```python
from build123d import *

# Parameters (mm, degrees)
SKETCH1_W                  = 85.725
SKETCH1_H                  = 38.1
BOSS_EXTRUDE1_DEPTH        = 12.7
F_1_2_0_5_DIAMETER_HOLE1_D = 12.7
F_1_4_CLEARANCE_HOLE1_D    = 6.7564


with BuildPart() as part:
    # Sketch1 → Boss-Extrude1 (new, symmetric)
    with BuildSketch(Plane(origin=(0, 0, 0), x_dir=(1, 0, 0), z_dir=(0, 1, 0))):
        Rectangle(SKETCH1_W, SKETCH1_H)
    extrude(amount=BOSS_EXTRUDE1_DEPTH, both=True)

    # 1/2 (0.5) Diameter Hole1 (through all)
    with Locations(Plane.XY.offset(19.05)):
        with Locations((30.1625, 0)):
            Hole(F_1_2_0_5_DIAMETER_HOLE1_D / 2)

    # 1/4 Clearance Hole1 (through all)
    with Locations(Plane(origin=(0, 12.7, 0), x_dir=(1, 0, 0), z_dir=(0, 1, 0))):
        with Locations((-33.3375, 0), (-1.5875, 0)):
            Hole(F_1_4_CLEARANCE_HOLE1_D / 2)


solid = part.part
```
Geometry: final body of the model. Coordinates: model frame, mm. Round coordinates to 2 decimals unless told otherwise and drop trailing zeros. Write each loop counter-clockwise with the first axis right and the second up, starting at its lowest first coordinate (ties: lowest second). Pieces come first, ordered by that corner, then holes. Notation, with made-up numbers: M 45.5,-20 L 101.5,-20 A29 cw 101.5,5 Z; hole C -32,9.25 d7. An arc over 180 degrees is marked long. Answer in a Markdown table with one row per item. Add a question column.
(1) Cut plane A-A, the plane y = 0. Return the cut outline in (x, z), then the cut area to 3 significant figures.
(2) Contact query for a flat-ended pin moving along its axis: pin 1 (4 mm diameter, centred on x = 26.5, y = 4, fed in from +Z). Output: stop coordinate, or through.
(3) Ray query, L1, parallel to X at y = 2, z = -0.5; L2, parallel to X at y = 5, z = 1; L3, parallel to X at y = -11.25, z = -1. Return the intervals inside material, ascending.
(4) Cut plane D-D, the plane z = 16.5. Return the cut outline in (x, y).
(5) Cut plane B-B, the plane z = 0. Return the cut outline in (x, y), then the cut area to 3 significant figures.
(6) Cut plane C-C, the plane y = -10.25. Return the cut outline in (x, z).
(7) Draft query along X for faces 1 (the face through (-1, -12.7, -5)), 2 (the face through (-0.86, -0.18, 3.3)), 3 (the face through (-42.862, 0, 0)), 4 (the face through (-29.963, -0.178, -0.149)). Return one class per face: pulls with the +X half, pulls with the -X half, needs draft (parallel to the pull), parting line crosses it, or undercut.
Established:
| question | item | result |
|---|---|---|
| 1 | outline | M -42.86,-19.05 L 23.81,-19.05 L 23.81,19.05 L -42.86,19.05 Z; M 36.51,-19.05 L 42.86,-19.05 L 42.86,19.05 L 36.51,19.05 Z; hole C -33.34,0 d6.76; hole C -1.59,0 d6.76 |
| 1 | area | 2,710 mm² |
| 2 | pin 1 | z = 19.05 |
| 3 | L1 | -42.86 to -36.68, -30 to -4.93, 1.75 to 24.14, 36.19 to 42.86 |
| 3 | L2 | -42.86 to -36.56, -30.11 to -4.81, 1.64 to 26.25, 34.08 to 42.86 |
| 3 | L3 | -42.86 to -36.56, -30.11 to -4.81, 1.64 to 42.86 |
| 4 | outline | M -42.86,-12.7 L 42.86,-12.7 L 42.86,12.7 L -42.86,12.7 Z; hole C 30.16,0 d12.7 |
| 5 | outline | M -42.86,-12.7 L -36.72,-12.7 L -36.72,12.7 L -42.86,12.7 Z; M -29.96,-12.7 L -4.97,-12.7 L -4.97,12.7 L -29.96,12.7 Z; M 1.79,-12.7 L 42.86,-12.7 L 42.86,12.7 L 1.79,12.7 Z; hole C 30.16,0 d12.7 |
| 5 | area | 1,710 mm² |
| 6 | outline | M -42.86,-19.05 L 42.86,-19.05 L 42.86,19.05 L -42.86,19.05 Z; hole C -33.34,0 d6.76; hole C -1.59,0 d6.76 |
| 7 | face 1 | needs draft |
| 7 | face 2 | undercut |
| 7 | face 3 | pulls with the -X half |
| 7 | face 4 | undercut |
